Solid Edge part; units mm, degrees
sketch "Sketch1" plane through (0, 0, 0) normal (0, 0, 1) x (1, 0, 0)
  line L0 (10, 2.5) -> (-10, 2.5)
  line L1 (-10, -2.5) -> (10, -2.5)
  arc A0 (-10, -2.5) -> (-10, 2.5) centre (-10, 0) cw
  arc A1 (10, 2.5) -> (10, -2.5) centre (10, 0) cw
  circle A2 centre (10, 0) radius 1.5
extrude "Protrusion1" add sketch "Sketch1" along normal blind 1.5
sketch "Sketch2" plane through (0, 0, 0.75) normal (0, 0, -1) x (1, 0, 0)
  line L0 (-14.75, 0) -> (-11.75, 0)
  arc A0 (-11.75, 0) -> (-14.75, 0) centre (-13.25, 0) cw
revolve "RevolvedProtrusion1" add sketch "Sketch2" angle 360 about axis through (-14.75, 0, 0.75) along (1, 0, 0)
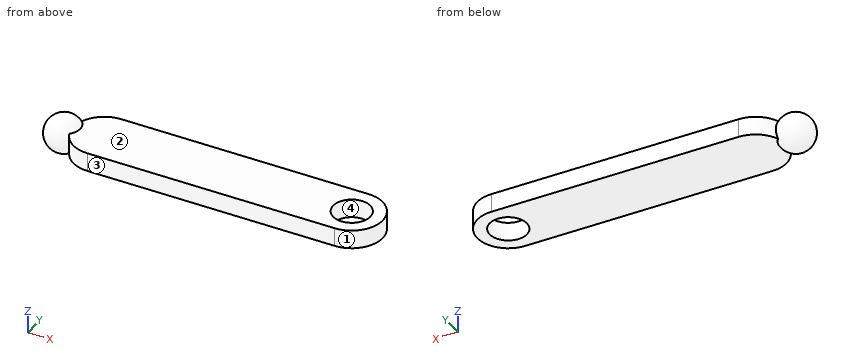
Design review of the part built by this model. Coordinates are the model's own, in mm. Face numbers are marked on the shaded views. Give positions to 0.01 mm unless a question says otherwise; leave off trailing zeros. Write each loop counter-clockwise with the first axis right and the second up, starting at its lowest first coordinate (ties: lowest second). Pieces come first, ordered by that corner, then holes. Notation, with made-up numbers: M 66.25,50.5 L 98.25,50.5 A17 ccw 98.25,78.5 Z; hole C -20.75,77.5 d3. An arc over 180 degrees is marked long. Answer as a JSON object with one key per item and string values. Group by question number.
1) We need section A-A (y = 0). Give the boundary of the cut face in (x, z), and give its area (3 significant figures).
2) Mouldability with a two-part tool opening along Y and no side actions: class the marked faces 1, 2, 3 and 4 as released by +Y, released by -Y, zero draft, split by the parting line, or undercut.
3) We need section C-C (x = 6.5). Give the boundary of the cut face in (y, z), and give its area (3 significant figures).
4) Clearance check with flat-ended pins moving along their axes: pin 1 Ø1.5 at (y, z) = (1, 0.5) entering from -X; pin 2 Ø3 at (x, y) = (7, -1) entering from +Z; pin 3 Ø1.5 at (x, y) = (-11.5, 1.5) entering from -Z. State where each tip first meets the part, or that it passes through.
5) We need section B-B (z = 0.4). Give the boundary of the cut face in (x, y), and give its area (3 significant figures).
6) For line 1 along Y through (x, z) = (10, 1.1); line 2 along Z through (x, y) = (-6, 0.6); line 3 along X through (y, z) = (0.95, 0.2), list the stretches that pass through material, from the lowest coordinate up.
Answer key:
{
 "1": {"outline": "M -11.95,0 L 8.5,0 L 8.5,1.5 L -11.95,1.5 A1.5 ccw long Z; M 11.5,0 L 12.5,0 L 12.5,1.5 L 11.5,1.5 Z", "area": "39.0 mm²"},
 "2": {"face 1": "split by the parting line", "face 2": "zero draft", "face 3": "released by -Y", "face 4": "undercut"},
 "3": {"outline": "M -2.5,0 L 2.5,0 L 2.5,1.5 L -2.5,1.5 Z", "area": "7.50 mm²"},
 "4": {"pin 1": "stops at x = -14.72", "pin 2": "stops at z = 1.5", "pin 3": "stops at z = 0"},
 "5": {"outline": "M -12.26,-1.07 A2.5 ccw -10,-2.5 L 10,-2.5 A2.5 ccw 10,2.5 L -10,2.5 A2.5 ccw -12.26,1.07 A1.46 ccw long Z; hole C 10,0 d3", "area": "118 mm²"},
 "6": {"line 1": "y = -2.5 to -1.5, 1.5 to 2.5", "line 2": "z = 0 to 1.5", "line 3": "x = -14.27 to 8.84, 11.16 to 12.31"}
}
